Autodesk Inventor part; units mm, degrees
ref_plane "YZ Plane" through (0, 0, 0) normal (1, 0, 0) x (0, 1, 0)
ref_plane "XZ Plane" through (0, 0, 0) normal (0, 1, 0) x (-1, 0, 0)
ref_plane "XY Plane" through (0, 0, 0) normal (0, 0, 1) x (1, 0, 0)
sketch "Эскиз1" plane through (0, 0, 0) normal (0, 0, 1) x (1, 0, 0)
  line L0 (-37, 0) -> (37, 0)
  line L1 (37, 0) -> (37, 82)
  line L2 (37, 82) -> (-37, 82)
  line L3 (-37, 82) -> (-37, 0)
  line L4 (-35, 0) -> (35, 0)
  line L5 (35, 0) -> (35, 80)
  line L6 (35, 80) -> (-35, 80)
  line L7 (-35, 80) -> (-35, 0)
  line L8 (0, -16.4) -> (0, 98.4)
  point P0 (0, 0)
  dimension "d0" = 70
  dimension "d1" = 80
  dimension "d2" = 2
  dimension "d3" = 2
  dimension "d4" = 2
extrude "Выдавливание1" add sketch "Эскиз1" along normal blind 30 contours L3 L2 L8 L6 L7 L0 | L2 L1 L0 L5 L6 L8
fillet "Сопряжение1" radius 15 2 edges at (36, 0, 0) (-36, 0, 0)
properties part number "выступ АКБ"
The model under review builds one solid part; all positions refer to its coordinate system, in mm. A direction names the side the tool comes from. Round coordinates to 2 decimals unless told otherwise and drop trailing zeros. Write each loop counter-clockwise with the first axis right and the second up, starting at its lowest first coordinate (ties: lowest second). Pieces come first, ordered by that corner, then holes. Notation, with made-up numbers: (-22, 52.25) -> (-15, 52.25) arc R12 ccw to (-15, 73.25) -> close; hole circle Ø9 at (-14.5, 66). An arc over 180 degrees is marked (long way). Answer as a JSON object with one key per item and string values.
1. We need section A-A on y = 61. State the section outline as (x, z) points.
Results found:
{"outline": "(-37, 0) -> (-35, 0) -> (-35, 30) -> (-37, 30) -> close; (35, 0) -> (37, 0) -> (37, 30) -> (35, 30) -> close"}
2. To check wall thickness, follow line 1 along X through (y, z) = (73, 9.25); line 2 along Y through (x, z) = (12, 14.5). State the ranges of each line that lie inside material, in increasing order.
Results found:
{"line 1": "x = -37 to -35, 35 to 37", "line 2": "y = 80 to 82"}
3. Machinability: for faces 4 (the face through (-35, 41, 15)), 5 (the face through (0, 81, 0)), which of the approach directions +Z, -Z, +X, -X, +Y, -Y give a long, thin tool a straight path to every point of the face, cutting with its end or side? Answer none if there is none.
Results found:
{"face 4": "+Z, -Z, -Y", "face 5": "-Z, +X, -X, +Y, -Y"}
4. We need section D-D on x = -11.5. State the section outline as (y, z) points.
Results found:
{"outline": "(80, 0) -> (82, 0) -> (82, 30) -> (80, 30) -> close"}
5. We need section C-C on y = 13. State the section outline as (x, z) points.
Results found:
{"outline": "(-37, 0.13) -> (-35, 0.13) -> (-35, 30) -> (-37, 30) -> close; (35, 0.13) -> (37, 0.13) -> (37, 30) -> (35, 30) -> close"}
6. Clearance check with a flat-ended pin moving along its axis: pin 1 (15 mm diameter, centred on x = 10.5, z = 13, fed in from -Y). State where the tip first meets the part, or that it passes through.
Results found:
{"pin 1": "stops at y = 80"}
7. We need section B-B on z = 20.5. State the section outline as (x, y) points, and give its area (3 significant figures).
Results found:
{"outline": "(-37, 0) -> (-35, 0) -> (-35, 80) -> (35, 80) -> (35, 0) -> (37, 0) -> (37, 82) -> (-37, 82) -> close", "area": "468 mm^2"}
8. The part is to be moulded in two halves that separate along X. For faces 1 (the face through (-37, 42, 15)), 2 (the face through (0, 80, 15)), 3 (the face through (1, 82, 15)), say which applies: pulls with the +X half, pulls with the -X half, needs draft (parallel to the pull), parting line crosses it, or undercut.
Results found:
{"face 1": "pulls with the -X half", "face 2": "undercut", "face 3": "needs draft"}
